from build123d import *

# Parameters (mm, degrees)
SKETCH1_W           = 30
SKETCH1_H           = 30
BOSS_EXTRUDE1_DEPTH = 60
CHAMFER1_SIZE       = 60
CHAMFER1_SIZE_2     = 29.263955314
SKETCH2_W           = 10
SKETCH2_H           = 30
CUT_EXTRUDE1_DEPTH  = 101


with BuildPart() as part:
    # Sketch1 → Boss-Extrude1 (new body)
    with BuildSketch(Plane(origin=(0, 0, 0), x_dir=(1, 0, 0), z_dir=(0, 1, 0))):
        with Locations((15, -15)):
            Rectangle(SKETCH1_W, SKETCH1_H)
    extrude(amount=BOSS_EXTRUDE1_DEPTH)

    # Chamfer1
    # the kernel refuses this chamfer: 60, 29.263955314 mm, written as the material it takes off along each edge
    with BuildSketch(Plane(origin=(30, 60, -155.415022708), x_dir=(0.01692389084982915, -0.999856780703368, 0), z_dir=(0, 0, 1)), Plane(origin=(185.415022708, 60, 30), x_dir=(0, -0.999856780703368, 0.01692389084982915), z_dir=(-1, 0, 0))) as chamfer1_piece_1:
        Polygon((CHAMFER1_SIZE * 0.999856780703, -CHAMFER1_SIZE * 0.0169238908498), (-CHAMFER1_SIZE_2 * 0.0169238908498, -CHAMFER1_SIZE_2 * 0.999856780702), (0, 0), align=None)
    extrude(amount=340.830045416, mode=Mode.SUBTRACT)

    # Sketch2 → Cut-Extrude1 (cut)
    with BuildSketch(Plane(origin=(0, 0, 0), x_dir=(1, 0, 0), z_dir=(0, 1, 0))):
        with Locations((25, -15)):
            Rectangle(SKETCH2_W, SKETCH2_H)
    extrude(amount=CUT_EXTRUDE1_DEPTH, mode=Mode.SUBTRACT)


solid = part.part
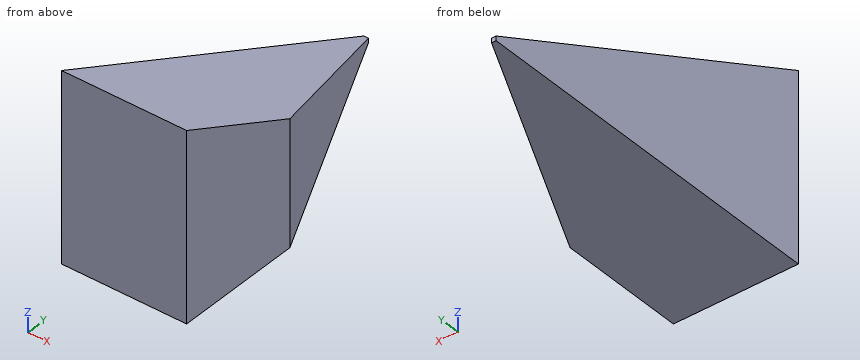
The model under review builds one solid part; all positions refer to its coordinate system, in mm. Round coordinates to 2 decimals unless told otherwise and drop trailing zeros. Loops run counter-clockwise (first coordinate to the right, second up) from the corner with the lowest first, then second, coordinate; pieces in that order, holes last. Notation, with made-up numbers: M 65.5,25.25 L 95.5,25.25 A8 cw 95.5,39.25 Z; hole C -16.75,56.5 d5. An arc over 180 degrees is marked long. Answer as CSV lines item,"result". Start each with the question number.
Item 1: Consider section A-A (z = 2.75). Write out the cut boundary in (x, y).
Item 2: Consider section B-B (y = 6.5). Write out the cut boundary in (x, z).
Item 3: Consider section D-D (z = 12.5). Write out the cut boundary in (x, y), then the cut area to 3 significant figures.
Item 4: Consider section C-C (x = 3). Write out the cut boundary in (y, z), then the cut area to 3 significant figures.
Item 5: Insertion check: P1, Ø10, axis at x = 14.5, y = 45.5, coming from the +Z side (3 decimals); P2, Ø12, axis at x = 11, z = 22.5, coming from the +Y side; P3, Ø1, axis at x = 3.5, y = 9.5, coming from the +Z side; P4, Ø4, axis at y = 36.5, z = 8, coming from the +X side. Each pin has a flat end and moves straight along its axis. Give the tip position at first contact, or say it passes through.
Item 6: Wall thickness on line 1 (Z direction, x = 5.5, y = 19.5); line 2 (Y direction, x = 5.5, z = 20); line 3 (Z direction, x = 14.75, y = 3.5): over which ranges is each line inside the solid? List them lowest first. Write a range as [from, to].
Answer:
1,outline,"M 0,0 L 20,0 L 20,20.5 L 2.75,55.87 L 0,55.87 Z"
2,outline,"M 0,0 L 20,0 L 20,26.83 L 0,26.83 Z"
3,outline,"M 0,0 L 20,0 L 20,20.5 L 12.5,35.88 L 0,35.88 Z"
3,area,"660 mm^2"
4,outline,"M 0,0 L 55.36,0 L 55.36,3 L 0,30 Z"
4,area,"913 mm^2"
5,P1,"passes through"
5,P2,"stops at y = 27.68"
5,P3,"stops at z = 25.61"
5,P4,"stops at x = 13.17"
6,line 1,"z = [0, 20.49]"
6,line 2,"y = [0, 20.5]"
6,line 3,"z = [0, 28.29]"
